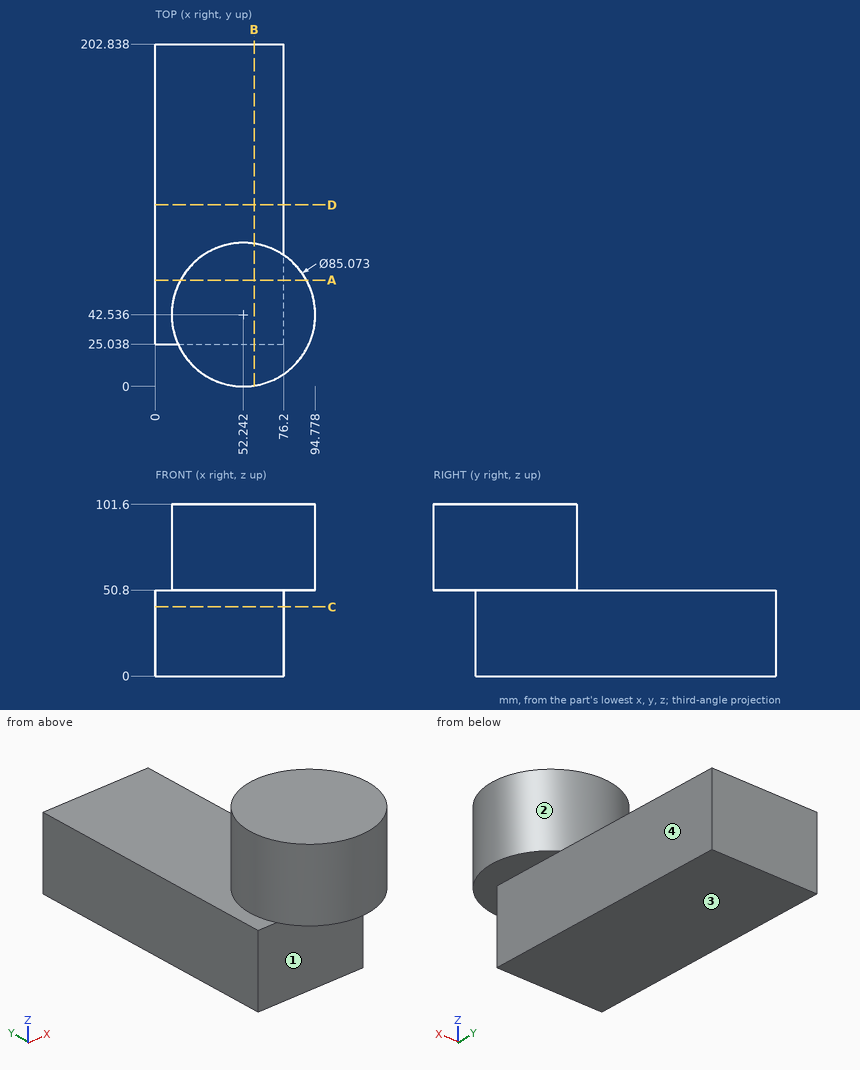
Check sheet for the drawn part. Datum: minimum x, y, z corner. Units: mm. A direction names the side the tool comes from. Round coordinates to 2 decimals unless told otherwise and drop trailing zeros. Loops run counter-clockwise (first coordinate to the right, second up) from the corner with the lowest first, then second, coordinate; pieces in that order, holes last. Notation, with made-up numbers: (-9.75, 37.5) -> (29.25, 37.5) arc R20 ccw to (29.25, 45.5) -> close; hole circle Ø4 at (-28.75, 65). An arc over 180 degrees is marked (long way). Put each result on its own line as item: value. Start each with the question number.
1. Gauge pin test, flat ends, axial feed: pin 1 (4 mm diameter, centred on x = 42, z = 76, fed in from -Y); pin 2 (1.5 mm diameter, centred on y = 80, z = 67.5, fed in from -X); pin 3 (6 mm diameter, centred on x = 48, y = 119, fed in from +Z). Record the tip position at first contact, or that the pin passes through.
2. Section check B-B (x = 58.5). Enter the section's corners in (y, z).
3. Section check C-C (z = 41). Enter the section's corners in (x, y), plus the area to 3 significant figures.
4. Section check A-A (y = 63). Enter the section's corners in (x, z), plus the area to 3 significant figures.
5. Section check D-D (y = 107.5). Enter the section's corners in (x, z).
6. Scan lines: probe 1 along Z at (x, y) = (24.5, 186); probe 2 along Y at (x, z) = (58, 49.5); probe 3 along X at (y, z) = (72, 11). Record each from-to range of solid material in increasing order.
7. Access from +Z, -Z, +X, -X, +Y, -Y to the whole of each face (thin tool, end or side, straight path). Record for the marked faces 1, 2, 3 and 4.
Findings:
1. pin 1: stops at y = 0.81
1. pin 2: stops at x = 30.76
1. pin 3: stops at z = 50.8
2. outline: (0.46, 50.8) -> (25.04, 50.8) -> (25.04, 0) -> (202.84, 0) -> (202.84, 50.8) -> (84.61, 50.8) -> (84.61, 101.6) -> (0.46, 101.6) -> close
3. outline: (0, 25.04) -> (76.2, 25.04) -> (76.2, 202.84) -> (0, 202.84) -> close
3. area: 13,500 mm^2
4. outline: (0, 0) -> (76.2, 0) -> (76.2, 50.8) -> (89.53, 50.8) -> (89.53, 101.6) -> (14.95, 101.6) -> (14.95, 50.8) -> (0, 50.8) -> close
4. area: 7,660 mm^2
5. outline: (0, 0) -> (76.2, 0) -> (76.2, 50.8) -> (0, 50.8) -> close
6. probe 1: z = 0 to 50.8
6. probe 2: y = 25.04 to 202.84
6. probe 3: x = 0 to 76.2
7. face 1: -Z, +X, -X, -Y
7. face 2: +Z
7. face 3: -Z, +X, -X, +Y, -Y
7. face 4: -Z, +X, +Y, -Y
